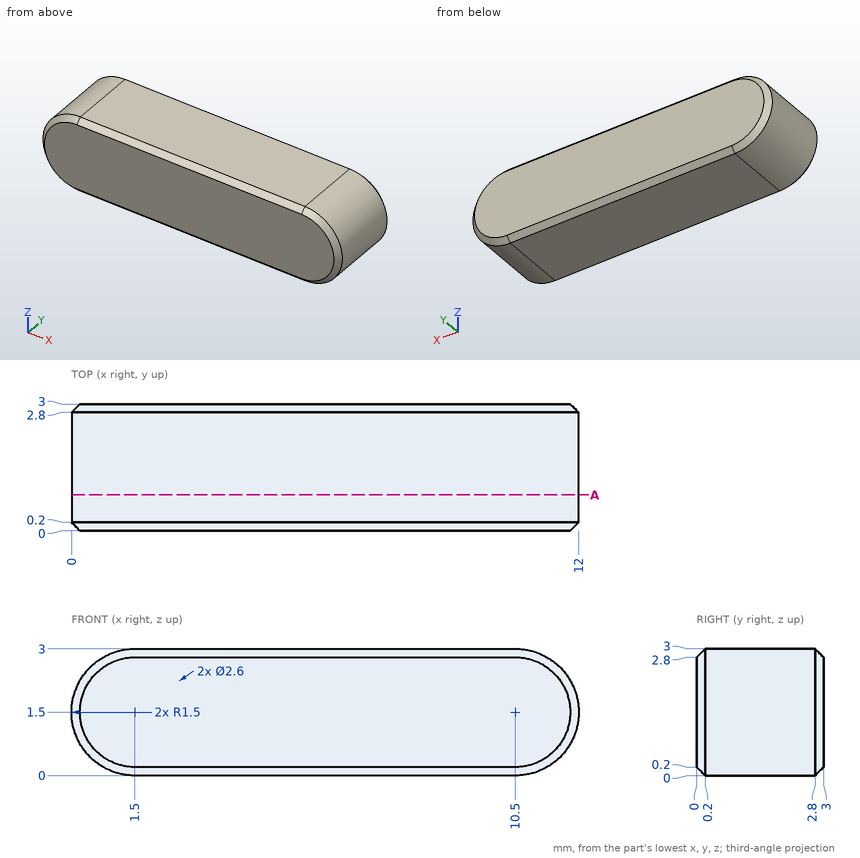
Study the drawing (mm; zero at the part's minimum x, y, z) and answer. Round coordinates to 2 decimals unless told otherwise and drop trailing zeros. Loops run counter-clockwise (first coordinate to the right, second up) from the corner with the lowest first, then second, coordinate; pieces in that order, holes last.
Q1. Given pin 1 Ø1 at (y, z) = (1.5, 0.5) entering from -X, flat-ended and moving along its own axis, determine where the tip first touches the part or whether it passes through.
Q2. Find the intervals of material crossed by line 1 (X direction, y = 0.9, z = 1.4); line 2 (Z direction, x = 11.25, y = 0.5); line 3 (X direction, y = 2.4, z = 0.7), in increasing order.
Q3. Section A-A, the plane y = 0.85 is taken. Determine the outline of the cut face in (x, z), then the cut area to 3 significant figures.
Completed:
1. pin 1: stops at x = 0.09
2. line 1: x = 0 to 12
2. line 2: z = 0.2 to 2.8
2. line 3: x = 0.23 to 11.77
3. outline: (1.5, 0) - (10.5, 0) arc R1.5 ccw to (10.5, 3) - (1.5, 3) arc R1.5 ccw to start
3. area: 34.1 mm2
